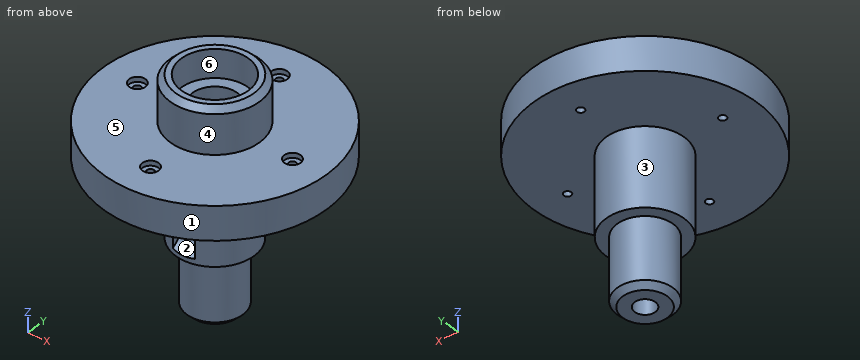
from build123d import *

# Parameters (mm, degrees)
SKETCH2_R                               = 30
CUT_EXTRUDE1_DEPTH                      = 10
CUT_EXTRUDE1_DEPTH_BACK                 = 10
CBORE_FOR_M6_HEX_HEAD_BOLT2_D           = 6.6
CBORE_FOR_M6_HEX_HEAD_BOLT2_CBORE_D     = 14.55
CBORE_FOR_M6_HEX_HEAD_BOLT2_CBORE_DEPTH = 4.38
CHAMFER1_SIZE                           = 5
M20X1_5_TAPPED_HOLE1_D                  = 18.5
M20X1_5_TAPPED_HOLE1_DEPTH              = 50
M20X1_5_TAPPED_HOLE1_TIP                = 5.557960726


with BuildPart() as part:
    # Sketch1 → Revolve1 (revolve)
    with BuildSketch(Plane(origin=(0, 0, 0), x_dir=(0, 0, -1), z_dir=(1, 0, 0))):
        Polygon((-200, 30), (-200, 40), (-160, 40), (-160, 100), (-130, 100), (-130, 35), (-60, 35), (-60, 25), (0, 25), (0, 0), (-155, 0), (-155, 20), (-175, 20), (-175, 30), align=None)
    revolve(axis=Axis((0, 0, 0), (0, 0, 1)))

    # Sketch2 → Cut-Extrude1 (cut, two sides)
    with BuildSketch(Plane(origin=(0, 0, 0), x_dir=(0, 0, -1), z_dir=(1, 0, 0))) as cut_extrude1_sk:
        with Locations((-90, -50)):
            Circle(SKETCH2_R)
    extrude(amount=CUT_EXTRUDE1_DEPTH, mode=Mode.SUBTRACT)
    extrude(cut_extrude1_sk.sketch, amount=-CUT_EXTRUDE1_DEPTH_BACK, mode=Mode.SUBTRACT)

    # CBORE for M6 Hex Head Bolt2 (through all)
    with Locations(Plane(origin=(0, 70, 160), x_dir=(0, 1, 0), z_dir=(0, 0, 1))):
        with Locations((0, 0), (-70, -70), (-140, 0), (-70, 70)):
            CounterBoreHole(CBORE_FOR_M6_HEX_HEAD_BOLT2_D / 2, CBORE_FOR_M6_HEX_HEAD_BOLT2_CBORE_D / 2, CBORE_FOR_M6_HEX_HEAD_BOLT2_CBORE_DEPTH)

    # Chamfer1
    chamfer1_edges = [part.edges().sort_by_distance(p)[0] for p in [
        (0, -40, 200),
        (0, -25, 0),
    ]]
    chamfer(chamfer1_edges, length=CHAMFER1_SIZE)

    # M20x1.5 Tapped Hole1
    with Locations(Plane(origin=(0, 0, 0), x_dir=(0, -1, 0), z_dir=(0, 0, -1))):
        with Locations((0, 0)):
            Hole(M20X1_5_TAPPED_HOLE1_D / 2, depth=M20X1_5_TAPPED_HOLE1_DEPTH)
            with Locations((0, 0, -(M20X1_5_TAPPED_HOLE1_DEPTH + M20X1_5_TAPPED_HOLE1_TIP / 2))):  # 118° drill point
                Cone(0, M20X1_5_TAPPED_HOLE1_D / 2, M20X1_5_TAPPED_HOLE1_TIP, mode=Mode.SUBTRACT)


solid = part.part
Check sheet for the modelled part. Datum: model origin and axes. Units: mm. Face numbers are marked on the shaded views. A direction names the side the tool comes from. Round coordinates to 2 decimals unless told otherwise and drop trailing zeros. Loops run counter-clockwise (first coordinate to the right, second up) from the corner with the lowest first, then second, coordinate; pieces in that order, holes last. Notation, with made-up numbers: (68, -27.5) -> (80, -27.5) arc R36 ccw to (80, 6.5) -> close; hole circle Ø10 at (-10, 3.5). An arc over 180 degrees is marked (long way). Put each result on its own line as item: value. Start each with the question number.
1. Draft check along X on the marked faces 4, 5 and 6. Enter one of: +X half, -X half, draft (parallel to the pull), parting line (faces both ways), or undercut.
2. Section check B-B (x = -70). Enter the section's corners in (y, z) (3 decimals), plus the area to 3 significant figures.
3. Access from +Z, -Z, +X, -X, +Y, -Y to the whole of each face (thin tool, end or side, straight path). Record for the marked faces 1, 2 and 3.
4. Scan lines: probe 1 along X at (y, z) = (0, 156.9) (3 decimals); probe 2 along X at (y, z) = (0, 161.75); probe 3 along X at (y, z) = (0, 184). Record each from-to range of solid material in increasing order.
5. Section check A-A (z = 137). Enter the section's corners in (x, y), plus the area to 3 significant figures.
6. Gauge pin test, flat ends, axial feed: pin 1 (2 mm diameter, centred on x = 46, y = 49, fed in from -Z); pin 2 (11.5 mm diameter, centred on x = 2.5, y = -71, fed in from +Z); pin 3 (16.5 mm diameter, centred on x = 0, y = 0, fed in from -Z). Record the tip position at first contact, or that the pin passes through.
7. Section check D-D (z = 13.5). Enter the section's corners in (x, y), plus the area to 3 significant figures.
Findings:
1. face 4: parting line
1. face 5: draft
1. face 6: undercut
2. outline: (-71.414, 130) -> (-3.3, 130) -> (-3.3, 155.62) -> (-7.275, 155.62) -> (-7.275, 160) -> (-71.414, 160) -> close; (3.3, 130) -> (71.414, 130) -> (71.414, 160) -> (7.275, 160) -> (7.275, 155.62) -> (3.3, 155.62) -> close
2. area: 4,050 mm^2
3. face 1: +Z, -Z
3. face 2: -Y
3. face 3: -Z
4. probe 1: x = -100 to -77.275, -62.725 to -20, 20 to 62.725, 77.275 to 100
4. probe 2: x = -40 to -20, 20 to 40
4. probe 3: x = -40 to -30, 30 to 40
5. outline: circle Ø200 at (0, 0); hole circle Ø6.6 at (-70, 0); hole circle Ø6.6 at (0, -70); hole circle Ø6.6 at (0, 70); hole circle Ø6.6 at (70, 0)
5. area: 31,300 mm^2
6. pin 1: stops at z = 130
6. pin 2: stops at z = 160
6. pin 3: stops at z = 50.6
7. outline: circle Ø50 at (0, 0); hole circle Ø18.5 at (0, 0)
7. area: 1,690 mm^2
